Source: CAD feature listing. Evaluate the final solid. Frame: model axes, mm. Face numbers are marked on the shaded views. A direction names the side the tool comes from. Coordinates: 2 decimals unless noted, no trailing zeros. Write each loop counter-clockwise with the first axis right and the second up, starting at its lowest first coordinate (ties: lowest second). Pieces come first, ordered by that corner, then holes. Notation, with made-up numbers: (78, 87.5) - (89, 87.5) arc R14 ccw to (89, 99.5) - close; hole circle Ø7 at (18.25, -33.75). An arc over 180 degrees is marked (long way). One line per item, written item: value.
from build123d import *

# Parameters (mm, degrees)
FILLET1_R           = 10
SKETCH12_R          = 3.05
SKETCH12_W          = 10
SKETCH12_H          = 10
BOSS_EXTRUDE4_DEPTH = 5
FILLET2_R           = 10
CUT_EXTRUDE5_REACH  = 198.959
SKETCH13_W          = 18
SKETCH13_H          = 100
REVOLVE2_ANGLE      = 180
BOSS_EXTRUDE5_DEPTH = 29
FILLET3_R           = 9
SKETCH15_W          = 42.078105567
SKETCH15_H          = 93.156211134
SKETCH15_W_2        = 21.921894433
SKETCH15_H_2        = 51
BOSS_EXTRUDE6_DEPTH = 3


with BuildPart() as part:
    # Sweep1: sweep along a path in r
    with BuildLine(Plane.XY) as sweep1_path:
        Line((29, -171), (-2, -171))
        ThreePointArc((-2, -171), (-23.213203436, -162.213203436), (-32, -141))
        Line((-32, -141), (-32, -40))
        Line((-32, -40), (29, -40))
    # Sketch11 → Sweep1 (sweep)
    with BuildSketch(Plane(origin=(29, 0, 0), x_dir=(0, 0, -1), z_dir=(1, 0, 0))):
        Polygon((0, -171), (0, -174), (29, -174), (29, -152.078105567), (26, -152.078105567), (26, -171), align=None)
    sweep(path=sweep1_path.line, transition=Transition.RIGHT)

    # Fillet1
    fillet1_edges = [part.edges().sort_by_distance(p)[0] for p in [
        (-23.213203436, -162.213203436, -26),
        (-32, -90.5, -26),
        (-1.5, -40, -26),
        (13.5, -171, -26),
    ]]
    fillet(fillet1_edges, radius=FILLET1_R)

    # Sketch12 → Boss-Extrude4 (add)
    # profile 1 of 2: a face of its own
    with BuildSketch(Plane.XY):
        with BuildLine():
            Line((29, 35), (5, 35))
            Line((5, 35), (-5, 35))
            ThreePointArc((-5, 35), (-26.575819403, 23.136416631), (-35, 0))
            Line((-35, 0), (-35, -141))
            ThreePointArc((-35, -141), (-26.372115214, -163.248595461), (-5, -173.86335345))
            Line((-5, -173.86335345), (-5, -184))
            Line((-5, -184), (5, -184))
            Line((5, -184), (5, -174))
            Line((5, -174), (29, -174))
            Line((29, -174), (29, 35))
        make_face()
        with Locations((0, -179)):
            Circle(SKETCH12_R, mode=Mode.SUBTRACT)
    # profile 2 of 2: a face of its own
    with BuildSketch(Plane.XY):
        with Locations((0, 40)):
            Rectangle(SKETCH12_W, SKETCH12_H)
        with Locations((0, 40)):
            Circle(SKETCH12_R, mode=Mode.SUBTRACT)
    extrude(amount=BOSS_EXTRUDE4_DEPTH)

    # Fillet2
    fillet2_edges = [part.edges().sort_by_distance(p)[0] for p in [
        (-23.213203436, -162.213203436, 0),
        (-32, -90.5, 0),
        (-1.5, -40, 0),
        (13.5, -171, 0),
    ]]
    fillet(fillet2_edges, radius=FILLET2_R)

    # Sketch13 → Cut-Extrude5 (cut, up to next)
    with BuildSketch(Plane.ZY.offset(35), mode=Mode.PRIVATE) as cut_extrude5_sk1:
        with Locations((-13, -126.5)):
            Rectangle(SKETCH13_W, SKETCH13_H)
    cut_extrude5_tool1 = extrude(cut_extrude5_sk1.sketch, amount=-CUT_EXTRUDE5_REACH, mode=Mode.PRIVATE) & part.part
    add(cut_extrude5_tool1.solids().sort_by_distance((-35, -126.5, -13))[0], mode=Mode.SUBTRACT)

    # Sketch14 → Revolve2 (revolve)
    with BuildSketch(Plane(origin=(0, 0, 0), x_dir=(0, 0, -1), z_dir=(1, 0, 0))):
        with BuildLine():
            Line((0, -35), (10, -35))
            ThreePointArc((10, -35), (21.313708499, -30.313708499), (26, -19))
            Line((26, -19), (23, -19))
            ThreePointArc((23, -19), (19.192388155, -28.192388155), (10, -32))
            Line((10, -32), (0, -32))
            Line((0, -32), (0, -35))
        make_face()
    revolve(axis=Axis((0, 0, -23), (0, 0, -1)), revolution_arc=REVOLVE2_ANGLE)

    # Sketch14<4> → Boss-Extrude5 (add, through all)
    with BuildSketch(Plane(origin=(0, 0, 0), x_dir=(0, 0, -1), z_dir=(1, 0, 0))):
        with BuildLine():
            Line((0, -32), (0, -35))
            Line((0, -35), (10, -35))
            ThreePointArc((10, -35), (21.313708499, -30.313708499), (26, -19))
            Line((26, -19), (23, -19))
            ThreePointArc((23, -19), (19.192388155, -28.192388155), (10, -32))
            Line((10, -32), (0, -32))
        make_face()
    boss_extrude5 = extrude(amount=BOSS_EXTRUDE5_DEPTH)

    # Mirror1: Boss-Extrude5 across plane
    add(boss_extrude5.mirror(Plane.ZX))

    # Fillet3
    fillet3_edges = [part.edges().sort_by_distance(p)[0] for p in [
        (-35, -37, -14.5),
    ]]
    fillet(fillet3_edges, radius=FILLET3_R)

    # Sketch15 → Boss-Extrude6 (add)
    with BuildSketch(Plane(origin=(0, 0, -29), x_dir=(-1, 0, 0), z_dir=(0, 0, -1))):
        with Locations((-7.960947217, -105.5)):
            Rectangle(SKETCH15_W, SKETCH15_H)
        with Locations((24.039052784, -102)):
            Rectangle(SKETCH15_W_2, SKETCH15_H_2)
    extrude(amount=-BOSS_EXTRUDE6_DEPTH)


solid = part.part
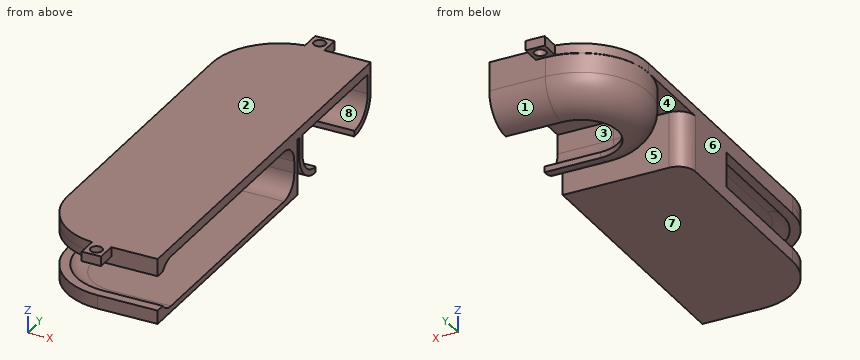
1) Contact query for flat-ended pins moving along their axis: P1, Ø1.5, axis at y = -180.5, z = 2, coming from the -X side; P2, Ø11, axis at x = 13.5, z = -7, coming from the +Y side; P3, Ø5, axis at y = -13, z = -16.5, coming from the +X side. Output: stop coordinate, or through.
Values found:
P1: x = -5
P2: y = 35
P3: x = -24.9
2) Section query C-C on y = -179. Output: boundary loops of the cut face in (x, z), then the cut area to 3 significant figures.
Values found:
outline: (-5, 0) - (-3.05, 0) - (-3.05, 5) - (-5, 5) - close; (3.05, 0) - (5, 0) - (5, 5) - (3.05, 5) - close
area: 19.5 mm2
3) Material intervals for line 1 (Y direction, x = 0, z = 3); line 2 (Y direction, x = 8, z = -7); line 3 (Y direction, x = -7.5, z = -3.5), sorted ascending.
Values found:
line 1: -184 to -182.05, -175.95 to 36.95, 43.05 to 45
line 2: -40.46 to -37, -35 to -32, 32 to 35
line 3: -173.54 to -168.05, -42.4 to -37, -34.19 to -31.11, 31.11 to 34.19
4) Reachability of the marked faces 4, 5, 6, 7 and 8 from +Z, -Z, +X, -X, +Y, -Y: full face, straight path, thin tool, end or side. Return the list, or none.
Values found:
face 4: -Z, -X
face 5: -Z, +X, -X
face 6: +Z, -Z, -X, +Y, -Y
face 7: -Z, +X, -X, +Y, -Y
face 8: +X
5) Section query B-B on x = 22.5. Output: boundary loops of the cut face in (y, z), then the cut area to 3 significant figures.
Values found:
outline: (-174, -29) - (-37, -29) - (-37, 0) - (-35, 0) - (-35, -10) arc R16 ccw to (-19, -26) - (-19, -23) arc R13 cw to (-32, -10) - (-32, 0) - (32, 0) - (32, -10) arc R13 cw to (19, -23) - (19, -26) arc R16 ccw to (35, -10) - (35, 5) - (-174, 5) - (-174, -4) - (-169, -4) arc R10 cw to (-161, 0) - (-50, 0) arc R10 cw to (-40, -10) - (-40, -16) arc R10 cw to (-50, -26) - (-161, -26) arc R10 cw to (-169, -22) - (-174, -22) - close
area: 1,830 mm2
6) Section query A-A on y = -95. Output: boundary loops of the cut face in (x, z), then the cut area to 3 significant figures.
Values found:
outline: (-35, -29) - (29, -29) - (29, -26) - (-22, -26) arc R10 cw to (-30, -22) - (-35, -22) - close; (-35, -4) - (-30, -4) arc R10 cw to (-22, 0) - (29, 0) - (29, 5) - (-35, 5) - close
area: 571 mm2
7) Draft query along Y for the marked faces 1, 2 and 3. Return one class per face: released by +Y, released by -Y, zero draft, split by the parting line, or undercut.
Values found:
face 1: released by +Y
face 2: zero draft
face 3: undercut
